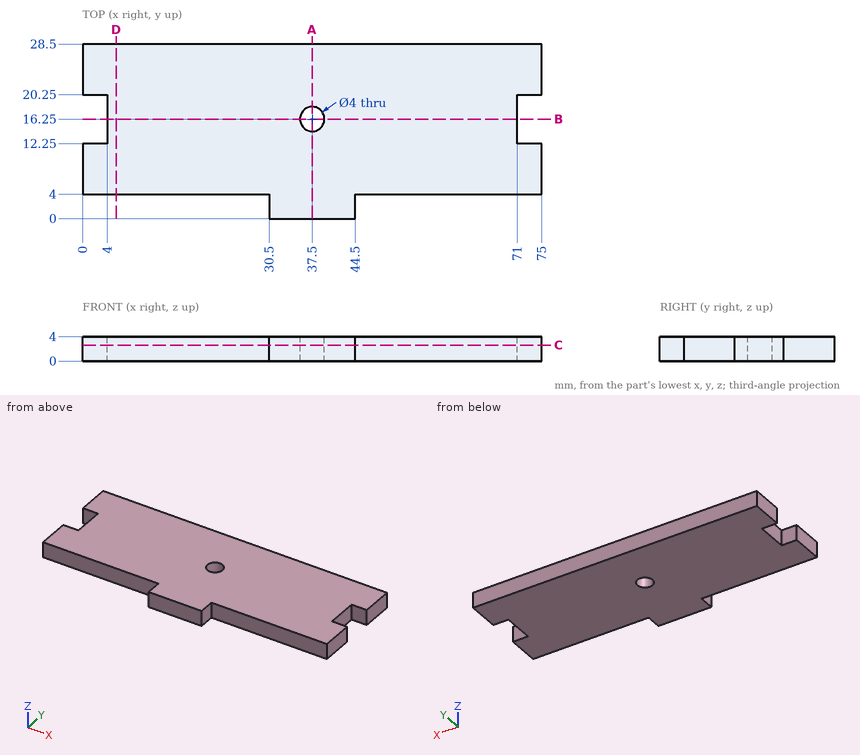
The drawing under review shows one solid part. Ordinate dimensions are in mm from its lowest x, y, z. Coordinates: 2 decimals unless noted, no trailing zeros. Order: outer loops, then holes, each group sorted by start corner. A loop starts at its lowest first (then second) coordinate and runs counter-clockwise, first axis right, second up. Notation, with made-up numbers: (-5.5, 43.5) - (2.5, 43.5) arc R9 cw to (2.5, 48.5) - close; hole circle Ø3 at (16.25, 17). An arc over 180 degrees is marked (long way). Put each result on its own line as item: value.
1) Insertion check: P1, Ø1.2, axis at x = 66, z = 1.5, coming from the -Y side; P2, Ø1.2, axis at y = 1.5, z = 1.5, coming from the -X side; P3, Ø2, axis at y = 17.5, z = 1.5, coming from the -X side. Each pin has a flat end and moves straight along its axis. Give the tip position at first contact, or say it passes through.
Response values:
P1: stops at y = 4
P2: stops at x = 30.5
P3: stops at x = 4
2) Take a section at A-A, the plane x = 37.5. Give the boundary of the cut face in (y, z).
Response values:
outline: (0, 0) - (14.25, 0) - (14.25, 4) - (0, 4) - close; (18.25, 0) - (28.5, 0) - (28.5, 4) - (18.25, 4) - close
3) Take a section at D-D, the plane x = 5.5. Give the boundary of the cut face in (y, z), and give its area (3 significant figures).
Response values:
outline: (4, 0) - (28.5, 0) - (28.5, 4) - (4, 4) - close
area: 98.0 mm²
4) Take a section at C-C, the plane z = 2.6. Give the boundary of the cut face in (x, y).
Response values:
outline: (0, 4) - (30.5, 4) - (30.5, 0) - (44.5, 0) - (44.5, 4) - (75, 4) - (75, 12.25) - (71, 12.25) - (71, 20.25) - (75, 20.25) - (75, 28.5) - (0, 28.5) - (0, 20.25) - (4, 20.25) - (4, 12.25) - (0, 12.25) - close; hole circle Ø4 at (37.5, 16.25)
5) Take a section at B-B, the plane y = 16.25. Give the boundary of the cut face in (x, z).
Response values:
outline: (4, 0) - (35.5, 0) - (35.5, 4) - (4, 4) - close; (39.5, 0) - (71, 0) - (71, 4) - (39.5, 4) - close
6) Wall thickness on L1, parallel to Y at x = 37.5, z = 2.7; L2, parallel to X at y = 13, z = 2.75; L3, parallel to X at y = 15, z = 2: over which ranges is each line inside the solid? List them lowest first. Write a range as from..to.
Response values:
L1: y = 0..14.25, 18.25..28.5
L2: x = 4..71
L3: x = 4..35.94, 39.06..71
